Geometry check sheet. Reference: the model listing, model coordinates, mm. A direction names the side the tool comes from. Give positions to 0.01 mm unless a question says otherwise; leave off trailing zeros. Write each loop counter-clockwise with the first axis right and the second up, starting at its lowest first coordinate (ties: lowest second). Pieces come first, ordered by that corner, then holes. Notation, with made-up numbers: M -36,35.25 L 19,35.25 A20 ccw 19,39.25 Z; hole C -3,59.5 d8. An arc over 180 degrees is marked long. One line per item, written item: value. Start each with the question number.
1. Tool access check on faces 1 (the face through (2, -32, 2)), 2 (the face through (23, -38, 2)), 3 (the face through (108, -16, 2)), 4 (the face through (71, -2, 2)), 5 (the face through (9, -28.995, 2)). Record the directions out of +Z, -Z, +X, -X, +Y, -Y that give a thin tool (end or side, any length) a straight path to the whole face; none if there is none.
2. Cross-section at A-A on y = -23. Record the cut outline in (x, z) (3 decimals).
3. Gauge pin test, flat ends, axial feed: pin 1 (1 mm diameter, centred on y = -1.5, z = 2, fed in from -X); pin 2 (1 mm diameter, centred on y = -1.5, z = 2, fed in from +X); pin 3 (1 mm diameter, centred on x = 48, z = 2.5, fed in from -Y) (3 decimals). Record the tip position at first contact, or that the pin passes through.
4. Cross-section at D-D on x = 30. Record the cut outline in (y, z) (3 decimals).
5. Cross-section at C-C on y = -33.5. Record the cut outline in (x, z) (3 decimals), then the cut area to 3 significant figures.
6. Scan lines: line 1 (X direction, y = -25, z = 2.8) (3 decimals); line 2 (X direction, y = -2.5, z = 0.5); line 3 (Y direction, x = 37.5, z = 2.1) (3 decimals). Record each from-to range of solid material in increasing order.
7. Cross-section at B-B on z = 1. Count the separate pieces of the cut face and the enclosed holes in it, then the cut area to 3 significant figures.
from build123d import *

# Parameters (mm, degrees)
SKETCH1_W           = 110
SKETCH1_H           = 40
BOSS_EXTRUDE1_DEPTH = 3.175
CUT_EXTRUDE5_REACH  = 5.175
SKETCH6_W           = 15
SKETCH6_H           = 3.175
SKETCH6_W_2         = 16
CUT_EXTRUDE6_REACH  = 5.175
SKETCH7_W           = 3.175
SKETCH7_H           = 4.825
SKETCH7_H_2         = 8
CUT_EXTRUDE7_REACH  = 5.175
SKETCH8_W           = 3.175
SKETCH8_H           = 8


with BuildPart() as part:
    # Sketch1 → Boss-Extrude1 (new body)
    with BuildSketch(Plane.XY):
        with Locations((55, -20)):
            Rectangle(SKETCH1_W, SKETCH1_H)
    extrude(amount=BOSS_EXTRUDE1_DEPTH)

    # Sketch6 → Cut-Extrude5 (cut, up to next)
    with BuildSketch(Plane(origin=(0, 0, 0), x_dir=(-1, 0, 0), z_dir=(0, 0, -1)), mode=Mode.PRIVATE) as cut_extrude5_sk1:
        with Locations((-102.5, -38.4125)):
            Rectangle(SKETCH6_W, SKETCH6_H)
    cut_extrude5_tool1 = extrude(cut_extrude5_sk1.sketch, amount=-CUT_EXTRUDE5_REACH, mode=Mode.PRIVATE) & part.part
    add(cut_extrude5_tool1.solids().sort_by_distance((102.5, -38.4125, 0))[0], mode=Mode.SUBTRACT)
    # Sketch6 → Cut-Extrude5 (cut, up to next)
    with BuildSketch(Plane(origin=(0, 0, 0), x_dir=(-1, 0, 0), z_dir=(0, 0, -1)), mode=Mode.PRIVATE) as cut_extrude5_sk2:
        with Locations((-55, -38.4125)):
            Rectangle(SKETCH6_W_2, SKETCH6_H)
    cut_extrude5_tool2 = extrude(cut_extrude5_sk2.sketch, amount=-CUT_EXTRUDE5_REACH, mode=Mode.PRIVATE) & part.part
    add(cut_extrude5_tool2.solids().sort_by_distance((55, -38.4125, 0))[0], mode=Mode.SUBTRACT)
    # Sketch6 → Cut-Extrude5 (cut, up to next)
    with BuildSketch(Plane(origin=(0, 0, 0), x_dir=(-1, 0, 0), z_dir=(0, 0, -1)), mode=Mode.PRIVATE) as cut_extrude5_sk3:
        with Locations((-31, -38.4125)):
            Rectangle(SKETCH6_W_2, SKETCH6_H)
    cut_extrude5_tool3 = extrude(cut_extrude5_sk3.sketch, amount=-CUT_EXTRUDE5_REACH, mode=Mode.PRIVATE) & part.part
    add(cut_extrude5_tool3.solids().sort_by_distance((31, -38.4125, 0))[0], mode=Mode.SUBTRACT)
    # Sketch6 → Cut-Extrude5 (cut, up to next)
    with BuildSketch(Plane(origin=(0, 0, 0), x_dir=(-1, 0, 0), z_dir=(0, 0, -1)), mode=Mode.PRIVATE) as cut_extrude5_sk4:
        with Locations((-7.5, -38.4125)):
            Rectangle(SKETCH6_W, SKETCH6_H)
    cut_extrude5_tool4 = extrude(cut_extrude5_sk4.sketch, amount=-CUT_EXTRUDE5_REACH, mode=Mode.PRIVATE) & part.part
    add(cut_extrude5_tool4.solids().sort_by_distance((7.5, -38.4125, 0))[0], mode=Mode.SUBTRACT)
    # Sketch6 → Cut-Extrude5 (cut, up to next)
    with BuildSketch(Plane(origin=(0, 0, 0), x_dir=(-1, 0, 0), z_dir=(0, 0, -1)), mode=Mode.PRIVATE) as cut_extrude5_sk5:
        with Locations((-79, -38.4125)):
            Rectangle(SKETCH6_W_2, SKETCH6_H)
    cut_extrude5_tool5 = extrude(cut_extrude5_sk5.sketch, amount=-CUT_EXTRUDE5_REACH, mode=Mode.PRIVATE) & part.part
    add(cut_extrude5_tool5.solids().sort_by_distance((79, -38.4125, 0))[0], mode=Mode.SUBTRACT)
    # Sketch6 → Cut-Extrude5 (cut, up to next)
    with BuildSketch(Plane(origin=(0, 0, 0), x_dir=(-1, 0, 0), z_dir=(0, 0, -1)), mode=Mode.PRIVATE) as cut_extrude5_sk6:
        with Locations((-55, -1.5875)):
            Rectangle(SKETCH6_W_2, SKETCH6_H)
    cut_extrude5_tool6 = extrude(cut_extrude5_sk6.sketch, amount=-CUT_EXTRUDE5_REACH, mode=Mode.PRIVATE) & part.part
    add(cut_extrude5_tool6.solids().sort_by_distance((55, -1.5875, 0))[0], mode=Mode.SUBTRACT)
    # Sketch6 → Cut-Extrude5 (cut, up to next)
    with BuildSketch(Plane(origin=(0, 0, 0), x_dir=(-1, 0, 0), z_dir=(0, 0, -1)), mode=Mode.PRIVATE) as cut_extrude5_sk7:
        with Locations((-79, -1.5875)):
            Rectangle(SKETCH6_W_2, SKETCH6_H)
    cut_extrude5_tool7 = extrude(cut_extrude5_sk7.sketch, amount=-CUT_EXTRUDE5_REACH, mode=Mode.PRIVATE) & part.part
    add(cut_extrude5_tool7.solids().sort_by_distance((79, -1.5875, 0))[0], mode=Mode.SUBTRACT)
    # Sketch6 → Cut-Extrude5 (cut, up to next)
    with BuildSketch(Plane(origin=(0, 0, 0), x_dir=(-1, 0, 0), z_dir=(0, 0, -1)), mode=Mode.PRIVATE) as cut_extrude5_sk8:
        with Locations((-102.5, -1.5875)):
            Rectangle(SKETCH6_W, SKETCH6_H)
    cut_extrude5_tool8 = extrude(cut_extrude5_sk8.sketch, amount=-CUT_EXTRUDE5_REACH, mode=Mode.PRIVATE) & part.part
    add(cut_extrude5_tool8.solids().sort_by_distance((102.5, -1.5875, 0))[0], mode=Mode.SUBTRACT)
    # Sketch6 → Cut-Extrude5 (cut, up to next)
    with BuildSketch(Plane(origin=(0, 0, 0), x_dir=(-1, 0, 0), z_dir=(0, 0, -1)), mode=Mode.PRIVATE) as cut_extrude5_sk9:
        with Locations((-7.5, -1.5875)):
            Rectangle(SKETCH6_W, SKETCH6_H)
    cut_extrude5_tool9 = extrude(cut_extrude5_sk9.sketch, amount=-CUT_EXTRUDE5_REACH, mode=Mode.PRIVATE) & part.part
    add(cut_extrude5_tool9.solids().sort_by_distance((7.5, -1.5875, 0))[0], mode=Mode.SUBTRACT)
    # Sketch6 → Cut-Extrude5 (cut, up to next)
    with BuildSketch(Plane(origin=(0, 0, 0), x_dir=(-1, 0, 0), z_dir=(0, 0, -1)), mode=Mode.PRIVATE) as cut_extrude5_sk10:
        with Locations((-31, -1.5875)):
            Rectangle(SKETCH6_W_2, SKETCH6_H)
    cut_extrude5_tool10 = extrude(cut_extrude5_sk10.sketch, amount=-CUT_EXTRUDE5_REACH, mode=Mode.PRIVATE) & part.part
    add(cut_extrude5_tool10.solids().sort_by_distance((31, -1.5875, 0))[0], mode=Mode.SUBTRACT)

    # Sketch7 → Cut-Extrude6 (cut, up to next)
    with BuildSketch(Plane(origin=(0, 0, 0), x_dir=(-1, 0, 0), z_dir=(0, 0, -1)), mode=Mode.PRIVATE) as cut_extrude6_sk1:
        with Locations((-108.4125, -34.4125)):
            Rectangle(SKETCH7_W, SKETCH7_H)
    cut_extrude6_tool1 = extrude(cut_extrude6_sk1.sketch, amount=-CUT_EXTRUDE6_REACH, mode=Mode.PRIVATE) & part.part
    add(cut_extrude6_tool1.solids().sort_by_distance((108.4125, -34.4125, 0))[0], mode=Mode.SUBTRACT)
    # Sketch7 → Cut-Extrude6 (cut, up to next)
    with BuildSketch(Plane(origin=(0, 0, 0), x_dir=(-1, 0, 0), z_dir=(0, 0, -1)), mode=Mode.PRIVATE) as cut_extrude6_sk2:
        with Locations((-108.4125, -20)):
            Rectangle(SKETCH7_W, SKETCH7_H_2)
    cut_extrude6_tool2 = extrude(cut_extrude6_sk2.sketch, amount=-CUT_EXTRUDE6_REACH, mode=Mode.PRIVATE) & part.part
    add(cut_extrude6_tool2.solids().sort_by_distance((108.4125, -20, 0))[0], mode=Mode.SUBTRACT)
    # Sketch7 → Cut-Extrude6 (cut, up to next)
    with BuildSketch(Plane(origin=(0, 0, 0), x_dir=(-1, 0, 0), z_dir=(0, 0, -1)), mode=Mode.PRIVATE) as cut_extrude6_sk3:
        with Locations((-108.4125, -5.5875)):
            Rectangle(SKETCH7_W, SKETCH7_H)
    cut_extrude6_tool3 = extrude(cut_extrude6_sk3.sketch, amount=-CUT_EXTRUDE6_REACH, mode=Mode.PRIVATE) & part.part
    add(cut_extrude6_tool3.solids().sort_by_distance((108.4125, -5.5875, 0))[0], mode=Mode.SUBTRACT)
    # Sketch7 → Cut-Extrude6 (cut, up to next)
    with BuildSketch(Plane(origin=(0, 0, 0), x_dir=(-1, 0, 0), z_dir=(0, 0, -1)), mode=Mode.PRIVATE) as cut_extrude6_sk4:
        with Locations((-1.5875, -20)):
            Rectangle(SKETCH7_W, SKETCH7_H_2)
    cut_extrude6_tool4 = extrude(cut_extrude6_sk4.sketch, amount=-CUT_EXTRUDE6_REACH, mode=Mode.PRIVATE) & part.part
    add(cut_extrude6_tool4.solids().sort_by_distance((1.5875, -20, 0))[0], mode=Mode.SUBTRACT)
    # Sketch7 → Cut-Extrude6 (cut, up to next)
    with BuildSketch(Plane(origin=(0, 0, 0), x_dir=(-1, 0, 0), z_dir=(0, 0, -1)), mode=Mode.PRIVATE) as cut_extrude6_sk5:
        with Locations((-1.5875, -34.4125)):
            Rectangle(SKETCH7_W, SKETCH7_H)
    cut_extrude6_tool5 = extrude(cut_extrude6_sk5.sketch, amount=-CUT_EXTRUDE6_REACH, mode=Mode.PRIVATE) & part.part
    add(cut_extrude6_tool5.solids().sort_by_distance((1.5875, -34.4125, 0))[0], mode=Mode.SUBTRACT)
    # Sketch7 → Cut-Extrude6 (cut, up to next)
    with BuildSketch(Plane(origin=(0, 0, 0), x_dir=(-1, 0, 0), z_dir=(0, 0, -1)), mode=Mode.PRIVATE) as cut_extrude6_sk6:
        with Locations((-1.5875, -5.5875)):
            Rectangle(SKETCH7_W, SKETCH7_H)
    cut_extrude6_tool6 = extrude(cut_extrude6_sk6.sketch, amount=-CUT_EXTRUDE6_REACH, mode=Mode.PRIVATE) & part.part
    add(cut_extrude6_tool6.solids().sort_by_distance((1.5875, -5.5875, 0))[0], mode=Mode.SUBTRACT)

    # Sketch8 → Cut-Extrude7 (cut, up to next)
    with BuildSketch(Plane(origin=(0, 0, 0), x_dir=(-1, 0, 0), z_dir=(0, 0, -1)), mode=Mode.PRIVATE) as cut_extrude7_sk1:
        with Locations((-38.0625, -24.995)):
            Rectangle(SKETCH8_W, SKETCH8_H)
    cut_extrude7_tool1 = extrude(cut_extrude7_sk1.sketch, amount=-CUT_EXTRUDE7_REACH, mode=Mode.PRIVATE) & part.part
    add(cut_extrude7_tool1.solids().sort_by_distance((38.0625, -24.995, 0))[0], mode=Mode.SUBTRACT)
    # Sketch8 → Cut-Extrude7 (cut, up to next)
    with BuildSketch(Plane(origin=(0, 0, 0), x_dir=(-1, 0, 0), z_dir=(0, 0, -1)), mode=Mode.PRIVATE) as cut_extrude7_sk2:
        with Locations((-89.2375, -24.995)):
            Rectangle(SKETCH8_W, SKETCH8_H)
    cut_extrude7_tool2 = extrude(cut_extrude7_sk2.sketch, amount=-CUT_EXTRUDE7_REACH, mode=Mode.PRIVATE) & part.part
    add(cut_extrude7_tool2.solids().sort_by_distance((89.2375, -24.995, 0))[0], mode=Mode.SUBTRACT)
    # Sketch8 → Cut-Extrude7 (cut, up to next)
    with BuildSketch(Plane(origin=(0, 0, 0), x_dir=(-1, 0, 0), z_dir=(0, 0, -1)), mode=Mode.PRIVATE) as cut_extrude7_sk3:
        with Locations((-9.2375, -24.995)):
            Rectangle(SKETCH8_W, SKETCH8_H)
    cut_extrude7_tool3 = extrude(cut_extrude7_sk3.sketch, amount=-CUT_EXTRUDE7_REACH, mode=Mode.PRIVATE) & part.part
    add(cut_extrude7_tool3.solids().sort_by_distance((9.2375, -24.995, 0))[0], mode=Mode.SUBTRACT)


solid = part.part
Report:
1. face 1: +Z, -Z, -X, -Y
1. face 2: +Z, -Z, -Y
1. face 3: +Z, -Z, +X
1. face 4: +Z, -Z, +Y
1. face 5: +Z, -Z
2. outline: M 3.175,0 L 7.65,0 L 7.65,3.175 L 3.175,3.175 Z; M 10.825,0 L 36.475,0 L 36.475,3.175 L 10.825,3.175 Z; M 39.65,0 L 87.65,0 L 87.65,3.175 L 39.65,3.175 Z; M 90.825,0 L 106.825,0 L 106.825,3.175 L 90.825,3.175 Z
3. pin 1: stops at x = 15
3. pin 2: stops at x = 95
3. pin 3: stops at y = -36.825
4. outline: M -36.825,0 L -3.175,0 L -3.175,3.175 L -36.825,3.175 Z
5. outline: M 3.175,0 L 106.825,0 L 106.825,3.175 L 3.175,3.175 Z
5. area: 329 mm^2
6. line 1: x = 0 to 7.65, 10.825 to 36.475, 39.65 to 87.65, 90.825 to 110
6. line 2: x = 15 to 23, 39 to 47, 63 to 71, 87 to 95
6. line 3: y = -36.825 to -28.995, -20.995 to -3.175
7. separate pieces: 1
7. enclosed holes: 3
7. area: 3,720 mm^2
